Part model, mm, in its own coordinate system. A direction names the side the tool comes from. Give positions to 0.01 mm unless a question says otherwise; leave off trailing zeros. Order: outer loops, then holes, each group sorted by start corner. A loop starts at its lowest first (then second) coordinate and runs counter-clockwise, first axis right, second up.
from build123d import *

# Parameters (mm, degrees)
SKETCH1_R           = 5
BOSS_EXTRUDE1_DEPTH = 20
SKETCH4_R           = 15
CUT_EXTRUDE1_DEPTH  = 2.5


with BuildPart() as part:
    # Sketch1 → Boss-Extrude1 (new body)
    with BuildSketch(Plane.XY):
        with BuildLine():
            Line((5.773502692, -10), (75, -10))
            ThreePointArc((75, -10), (85, 0), (75, 10))
            Line((75, 10), (0, 10))
            ThreePointArc((0, 10), (-5, 8.660254038), (-8.660254038, 5))
            Line((-8.660254038, 5), (-31.160254038, -33.97114317))
            ThreePointArc((-31.160254038, -33.97114317), (-27.5, -47.631397208), (-13.839745962, -43.97114317))
            Line((-13.839745962, -43.97114317), (5.773502692, -10))
        make_face()
        with Locations((-22.5, -38.97114317)):
            Circle(SKETCH1_R, mode=Mode.SUBTRACT)
        Circle(SKETCH1_R, mode=Mode.SUBTRACT)
        with Locations((75, 0)):
            Circle(SKETCH1_R, mode=Mode.SUBTRACT)
    extrude(amount=BOSS_EXTRUDE1_DEPTH)

    # Sketch4 → Cut-Extrude1 (cut, symmetric)
    with BuildSketch(Plane(origin=(0, 0, 10), x_dir=(-1, 0, 0), z_dir=(0, 0, -1))):
        with Locations((22.5, -38.97114317)):
            Circle(SKETCH4_R)
    extrude(amount=CUT_EXTRUDE1_DEPTH, both=True, mode=Mode.SUBTRACT)


solid = part.part
Item 1: Pull direction Z, two halves, no side cores. Call faces 1 (the face through (-15.133, -25.905, 9.965)), 2 (the face through (17, -8, 20)), 3 (the face through (79.619, -1.915, 9.86)): released by +Z, released by -Z, zero draft, split by the parting line, or undercut.
Item 2: Which spindle directions (+Z, -Z, +X, -X, +Y, -Y) get a long thin tool onto all of the face, cutting with end or side? Do faces 4 (the face through (40, -10, 10)), 5 (the face through (-19.75, -14.21, 9.86)). Say none if no direction does.
Item 3: Drill centre lines: probe 1 along X at (y, z) = (4.5, 14.5); probe 2 along Z at (x, y) = (-27.5, -28.5); probe 3 along Y at (x, z) = (75, 6.25). Where is each one in solid material? Low to high.
Item 4: Band-saw the part on A-A on y = 0. List the corners of the cut face in (x, z).
Item 5: Band-saw the part on C-C on y = -37.5. List the corners of the cut face in (x, z), plus the area to 3 significant figures.
Item 6: Drop flat-ended pins along their axis: P1, Ø3, axis at y = -26, z = 2.5, coming from the -X side; P2, Ø12, axis at y = -22, z = 13, coming from the +X side; P3, Ø2, axis at y = -22, z = 11, coming from the -X side. Give the stop position or say it passes through.
Item 7: Band-saw the part on D-D on x = -22.5. List the corners of the cut face in (y, z).
Item 8: Band-saw the part on B-B on z = 8.75. List the corners of the cut face in (x, y), plus the area to 3 significant figures.
Working result:
1. face 1: undercut
1. face 2: released by +Z
1. face 3: zero draft
2. face 4: +Z, -Z, +X, -Y
2. face 5: +Z, -Z, -X, +Y
3. probe 1: x = -8.95 to -2.18, 2.18 to 72.82, 77.18 to 83.93
3. probe 2: z = 0 to 7.5, 12.5 to 20
3. probe 3: y = -10 to -5, 5 to 10
4. outline: (-11.55, 0) - (-5, 0) - (-5, 20) - (-11.55, 20) - close; (5, 0) - (70, 0) - (70, 20) - (5, 20) - close; (80, 0) - (85, 0) - (85, 20) - (80, 20) - close
5. outline: (-32.39, 0) - (-27.28, 0) - (-27.28, 7.5) - (-32.39, 7.5) - close; (-32.39, 12.5) - (-27.28, 12.5) - (-27.28, 20) - (-32.39, 20) - close; (-17.72, 0) - (-10.1, 0) - (-10.1, 7.5) - (-17.72, 7.5) - close; (-17.72, 12.5) - (-10.1, 12.5) - (-10.1, 20) - (-17.72, 20) - close
5. area: 191 mm2
6. P1: stops at x = -27.42
6. P2: stops at x = 2.31
6. P3: stops at x = -24.83
7. outline: (-48.97, 0) - (-43.97, 0) - (-43.97, 7.5) - (-48.97, 7.5) - close; (-48.97, 12.5) - (-43.97, 12.5) - (-43.97, 20) - (-48.97, 20) - close; (-33.97, 0) - (-18.97, 0) - (-18.97, 20) - (-33.97, 20) - (-33.97, 12.5) - (-23.97, 12.5) - (-23.97, 7.5) - (-33.97, 7.5) - close
8. outline: (-25.57, -24.29) arc R15 cw to (-8.25, -34.29) - (5.77, -10) - (75, -10) arc R10 ccw to (75, 10) - (0, 10) arc R10 ccw to (-8.66, 5) - close; hole circle Ø10 at (0, 0); hole circle Ø10 at (75, 0)
8. area: 2,120 mm2
